from build123d import *

# Parameters (mm, degrees)
SKETCH_R  = 0.9
SKETCH_W  = 13.6
SKETCH_H  = 13.6
PAD_DEPTH = 1.3


with BuildPart() as part:
    # Sketch → Pad (new body)
    with BuildSketch(Plane.XY):
        with BuildLine():
            ThreePointArc((0, 18.6), (-3.535534, 17.135534), (-5, 13.6))
            Line((-5, 13.6), (-5, -57))
            ThreePointArc((-5, -57), (-3.535534, -60.535534), (0, -62))
            Line((0, -62), (108.6, -62))
            ThreePointArc((108.6, -62), (112.135534, -60.535534), (113.6, -57))
            Line((113.6, -57), (113.6, 13.6))
            ThreePointArc((113.6, 13.6), (112.135534, 17.135534), (108.6, 18.6))
            Line((108.6, 18.6), (0, 18.6))
        make_face()
        with Locations((92.3, -40.7)):
            Circle(SKETCH_R, mode=Mode.SUBTRACT)
        with Locations((54.3, -40.7)):
            Circle(SKETCH_R, mode=Mode.SUBTRACT)
        with Locations((16.3, -40.7)):
            Circle(SKETCH_R, mode=Mode.SUBTRACT)
        with Locations((16.3, -2.7)):
            Circle(SKETCH_R, mode=Mode.SUBTRACT)
        with Locations((54.3, -2.7)):
            Circle(SKETCH_R, mode=Mode.SUBTRACT)
        with Locations((92.3, -2.7)):
            Circle(SKETCH_R, mode=Mode.SUBTRACT)
        with Locations((6.8, 6.8)):
            Rectangle(SKETCH_W, SKETCH_H, mode=Mode.SUBTRACT)
        with Locations((25.8, 6.8)):
            Rectangle(SKETCH_W, SKETCH_H, mode=Mode.SUBTRACT)
        with Locations((44.8, 6.8)):
            Rectangle(SKETCH_W, SKETCH_H, mode=Mode.SUBTRACT)
        with Locations((63.8, 6.8)):
            Rectangle(SKETCH_W, SKETCH_H, mode=Mode.SUBTRACT)
        with Locations((82.8, 6.8)):
            Rectangle(SKETCH_W, SKETCH_H, mode=Mode.SUBTRACT)
        with Locations((101.8, 6.8)):
            Rectangle(SKETCH_W, SKETCH_H, mode=Mode.SUBTRACT)
        with Locations((6.8, -12.2)):
            Rectangle(SKETCH_W, SKETCH_H, mode=Mode.SUBTRACT)
        with Locations((25.8, -12.2)):
            Rectangle(SKETCH_W, SKETCH_H, mode=Mode.SUBTRACT)
        with Locations((44.8, -12.2)):
            Rectangle(SKETCH_W, SKETCH_H, mode=Mode.SUBTRACT)
        with Locations((63.8, -12.2)):
            Rectangle(SKETCH_W, SKETCH_H, mode=Mode.SUBTRACT)
        with Locations((82.8, -12.2)):
            Rectangle(SKETCH_W, SKETCH_H, mode=Mode.SUBTRACT)
        with Locations((101.8, -12.2)):
            Rectangle(SKETCH_W, SKETCH_H, mode=Mode.SUBTRACT)
        with Locations((6.8, -31.2)):
            Rectangle(SKETCH_W, SKETCH_H, mode=Mode.SUBTRACT)
        with Locations((25.8, -31.2)):
            Rectangle(SKETCH_W, SKETCH_H, mode=Mode.SUBTRACT)
        with Locations((44.8, -31.2)):
            Rectangle(SKETCH_W, SKETCH_H, mode=Mode.SUBTRACT)
        with Locations((63.8, -31.2)):
            Rectangle(SKETCH_W, SKETCH_H, mode=Mode.SUBTRACT)
        with Locations((82.8, -31.2)):
            Rectangle(SKETCH_W, SKETCH_H, mode=Mode.SUBTRACT)
        with Locations((101.8, -31.2)):
            Rectangle(SKETCH_W, SKETCH_H, mode=Mode.SUBTRACT)
        with Locations((6.8, -50.2)):
            Rectangle(SKETCH_W, SKETCH_H, mode=Mode.SUBTRACT)
        with Locations((25.8, -50.2)):
            Rectangle(SKETCH_W, SKETCH_H, mode=Mode.SUBTRACT)
        with Locations((44.8, -50.2)):
            Rectangle(SKETCH_W, SKETCH_H, mode=Mode.SUBTRACT)
        with Locations((63.8, -50.2)):
            Rectangle(SKETCH_W, SKETCH_H, mode=Mode.SUBTRACT)
        with Locations((82.8, -50.2)):
            Rectangle(SKETCH_W, SKETCH_H, mode=Mode.SUBTRACT)
        with Locations((101.8, -50.2)):
            Rectangle(SKETCH_W, SKETCH_H, mode=Mode.SUBTRACT)
    extrude(amount=PAD_DEPTH)


solid = part.part
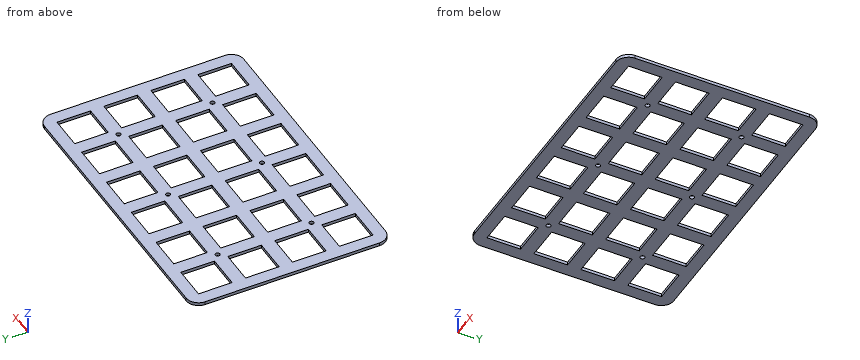
Geometry check sheet. Reference: the model listing, model coordinates, mm. Give positions to 0.01 mm unless a question says otherwise; leave off trailing zeros. Loops run counter-clockwise (first coordinate to the right, second up) from the corner with the lowest first, then second, coordinate; pieces in that order, holes last.
(1) Section check B-B on x = 81.5. Record the cut outline in (y, z).
From the geometry:
outline: (-62, 0) - (-57, 0) - (-57, 1.3) - (-62, 1.3) - close; (-43.4, 0) - (-38, 0) - (-38, 1.3) - (-43.4, 1.3) - close; (-24.4, 0) - (-19, 0) - (-19, 1.3) - (-24.4, 1.3) - close; (-5.4, 0) - (0, 0) - (0, 1.3) - (-5.4, 1.3) - close; (13.6, 0) - (18.6, 0) - (18.6, 1.3) - (13.6, 1.3) - close
(2) Section check A-A on y = -55.5. Record the cut outline in (x, z).
From the geometry:
outline: (-5, 0) - (0, 0) - (0, 1.3) - (-5, 1.3) - close; (13.6, 0) - (19, 0) - (19, 1.3) - (13.6, 1.3) - close; (32.6, 0) - (38, 0) - (38, 1.3) - (32.6, 1.3) - close; (51.6, 0) - (57, 0) - (57, 1.3) - (51.6, 1.3) - close; (70.6, 0) - (76, 0) - (76, 1.3) - (70.6, 1.3) - close; (89.6, 0) - (95, 0) - (95, 1.3) - (89.6, 1.3) - close; (108.6, 0) - (113.6, 0) - (113.6, 1.3) - (108.6, 1.3) - close
(3) Thickness scan on L1, parallel to Y at x = 92.3, z = 0.3; L2, parallel to Y at x = 12.5, z = 0.6; L3, parallel to X at y = -40.7, z = 0.9. Record the ranges inside material, lowest first.
From the geometry:
L1: y = -62 to -41.6, -39.8 to -3.6, -1.8 to 18.6
L2: y = -62 to -57, -43.4 to -38, -24.4 to -19, -5.4 to 0, 13.6 to 18.6
L3: x = -5 to 15.4, 17.2 to 53.4, 55.2 to 91.4, 93.2 to 113.6
(4) Section check C-C on z = 0.7. Count the separate pieces of the cut face and the enclosed holes in it, then the cut area to 3 significant figures.
From the geometry:
separate pieces: 1
enclosed holes: 30
area: 5,080 mm2
